Part print with two shaded views. Sizes in mm from the minimum x, y, z corner. Round coordinates to 2 decimals unless told otherwise and drop trailing zeros. Order: outer loops, then holes, each group sorted by start corner. A loop starts at its lowest first (then second) coordinate and runs counter-clockwise, first axis right, second up. Notation, with made-up numbers: (30.25, -3) -> (81.25, -3) arc R20 ccw to (81.25, 35) -> close; hole circle Ø2 at (84.25, 13.5). An arc over 180 degrees is marked (long way). Put each result on its own line as item: value. Start each with the question number.
Q1. Probe L1, parallel to Y at x = 3.14, z = 1.15; L2, parallel to X at y = 2.5, z = 0.8; L3, parallel to Y at x = 2, z = 1.8. List the from-to ranges inside material, lowest first.
Q2. Cut at A-A, the plane x = 3.14. List the corners of the cut face in (y, z).
Q3. Pull direction X, two halves, no side cores. Call the marked faces 1, 2 and 3: released by +X, released by -X, zero draft, split by the parting line, or undercut.
Q4. Flat gauge pins, fed straight in: P1, Ø1, axis at x = 4.5, z = 1, coming from the -Y side; P2, Ø2, axis at x = 1, z = 1, coming from the +Y side. Where does each tip first touch, or does it go through?
Q5. Cut at C-C, the plane z = 2.3. List the corners of the cut face in (x, y), and give its area (3 significant figures).
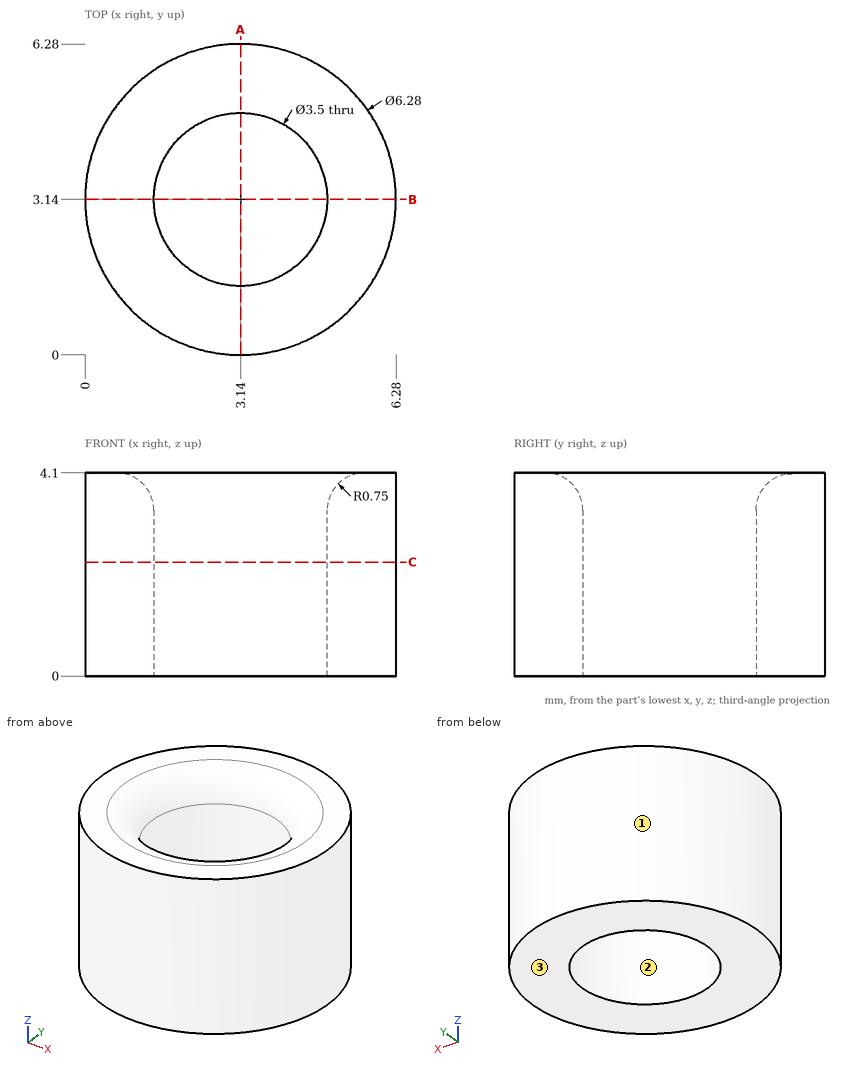
Ans:
1. L1: y = 0 to 1.39, 4.89 to 6.28
1. L2: x = 0.07 to 1.51, 4.77 to 6.21
1. L3: y = 0.21 to 1.81, 4.47 to 6.07
2. outline: (0, 0) -> (1.39, 0) -> (1.39, 3.35) arc R0.75 ccw to (0.64, 4.1) -> (0, 4.1) -> close; (4.89, 0) -> (6.28, 0) -> (6.28, 4.1) -> (5.64, 4.1) arc R0.75 ccw to (4.89, 3.35) -> close
3. face 1: split by the parting line
3. face 2: undercut
3. face 3: zero draft
4. P1: stops at y = 0.12
4. P2: stops at y = 6.07
5. outline: circle Ø6.28 at (3.14, 3.14); hole circle Ø3.5 at (3.14, 3.14)
5. area: 21.4 mm^2
